```python
from build123d import *

# Parameters (mm, degrees)
SKETCH_1_W          = 60
SKETCH_1_H          = 108
EXTRUDE_1_DEPTH     = 1
SKETCH_4_R          = 1.4
CUT_EXTRUDE_2_DEPTH = 10
SKETCH_9_R          = 1.6
CUT_EXTRUDE_5_DEPTH = 62.781874365
FILLET_1_R          = 5


with BuildPart() as part:
    # ｽｹｯﾁ1 → ﾎﾞｽ - 押し出し1 (new body)
    with BuildSketch(Plane.XY):
        Rectangle(SKETCH_1_W, SKETCH_1_H)
    extrude(amount=EXTRUDE_1_DEPTH)

    # ｽｹｯﾁ4 → ｶｯﾄ - 押し出し2 (cut)
    with BuildSketch(Plane.XY.offset(1)):
        with Locations((-24.5, 3)):
            Circle(SKETCH_4_R)
        with Locations((-24.5, -39)):
            Circle(SKETCH_4_R)
        with Locations((24.5, 3)):
            Circle(SKETCH_4_R)
        with Locations((24.5, -39)):
            Circle(SKETCH_4_R)
    extrude(amount=-CUT_EXTRUDE_2_DEPTH, mode=Mode.SUBTRACT)

    # ｽｹｯﾁ9 → ｶｯﾄ - 押し出し5 (cut, through all)
    with BuildSketch(Plane.XY.offset(1)):
        with Locations((25, 49)):
            Circle(SKETCH_9_R)
        with Locations((-25, 49)):
            Circle(SKETCH_9_R)
        with Locations((-25, -49)):
            Circle(SKETCH_9_R)
        with Locations((25, -49)):
            Circle(SKETCH_9_R)
    extrude(amount=-CUT_EXTRUDE_5_DEPTH, mode=Mode.SUBTRACT)

    # ﾌｨﾚｯﾄ1
    fillet_1_edges = [part.edges().sort_by_distance(p)[0] for p in [
        (30, -54, 0.5),
        (-30, -54, 0.5),
        (-30, 54, 0.5),
        (30, 54, 0.5),
    ]]
    fillet(fillet_1_edges, radius=FILLET_1_R)


solid = part.part
```
Check sheet for the modelled part. Datum: model origin and axes. Units: mm. Coordinates: 2 decimals unless noted, no trailing zeros. Order: outer loops, then holes, each group sorted by start corner. A loop starts at its lowest first (then second) coordinate and runs counter-clockwise, first axis right, second up. Notation, with made-up numbers: (34.5, 27) -> (58.5, 27) arc R3 ccw to (58.5, 32) -> close; hole circle Ø6 at (10, 21.5). An arc over 180 degrees is marked (long way). Write item = value, one per line. Start each with the question number.
1) Material ranges on L1, parallel to Y at x = 24.5, z = 0.6; L2, parallel to X at y = 48, z = 0.4; L3, parallel to X at y = -38, z = 0.1, recorded low to high.
2) Cross-section at A-A (y = -39). Enter the section's corners in (x, z), then the cut area to 3 significant figures.
3) Mould release check, pull along Y, two halves, no side actions. Record for faces 1 (the cylindrical face through (-28.57, -52.5, 0.51)), 2 (the cylindrical face through (-24.68, -37.61, 0.51)), 3 (the flat face through (0, 1, 1)): +Y half, -Y half, draft (parallel to the pull), parting line (faces both ways), or undercut.
Ans:
q1.L1 = -54 to -50.52, -47.48 to -40.4, -37.6 to 1.6, 4.4 to 47.48, 50.52 to 54
q1.L2 = -30 to -26.25, -23.75 to 23.75, 26.25 to 30
q1.L3 = -30 to -25.48, -23.52 to 23.52, 25.48 to 30
q2.outline = (-30, 0) -> (-25.9, 0) -> (-25.9, 1) -> (-30, 1) -> close; (-23.1, 0) -> (23.1, 0) -> (23.1, 1) -> (-23.1, 1) -> close; (25.9, 0) -> (30, 0) -> (30, 1) -> (25.9, 1) -> close
q2.area = 54.4 mm²
q3.face_1 = -Y half
q3.face_2 = undercut
q3.face_3 = draft
